```python
from build123d import *

# Parameters (mm, degrees)
SKETCH1_R           = 7.75
SKETCH1_R_2         = 1.524
BOSS_EXTRUDE1_DEPTH = 3.048
BOSS_EXTRUDE2_DEPTH = 25.4
CUT_EXTRUDE1_DEPTH  = 35.925


with BuildPart() as part:
    # Sketch1 → Boss-Extrude1 (new body)
    with BuildSketch(Plane(origin=(0, 0, 0), x_dir=(1, 0, 0), z_dir=(0, 1, 0))):
        with BuildLine():
            Line((25.4, 12.7), (25.4, -12.7))
            Line((25.4, -12.7), (22.225, -12.7))
            Line((22.225, -12.7), (3.175, -17.4625))
            Line((3.175, -17.4625), (0, -17.4625))
            ThreePointArc((0, -17.4625), (-1.398490879, -17.111633495), (-2.465718563, -16.142144397))
            Line((-2.465718563, -16.142144397), (-9.155410697, -6.097413793))
            ThreePointArc((-9.155410697, -6.097413793), (-11, 0), (-9.155410697, 6.097413793))
            Line((-9.155410697, 6.097413793), (-2.465718563, 16.142144397))
            ThreePointArc((-2.465718563, 16.142144397), (-1.398490879, 17.111633495), (0, 17.4625))
            Line((0, 17.4625), (3.175, 17.4625))
            Line((3.175, 17.4625), (22.225, 12.7))
            Line((22.225, 12.7), (25.4, 12.7))
        make_face()
        Circle(SKETCH1_R, mode=Mode.SUBTRACT)
        with Locations((0, 14.5)):
            Circle(SKETCH1_R_2, mode=Mode.SUBTRACT)
        with Locations((0, -14.5)):
            Circle(SKETCH1_R_2, mode=Mode.SUBTRACT)
    extrude(amount=BOSS_EXTRUDE1_DEPTH)

    # Sketch2 → Boss-Extrude2 (add)
    with BuildSketch(Plane(origin=(0, 3.048, 0), x_dir=(1, 0, 0), z_dir=(0, 1, 0))):
        Polygon((3.175, 17.4625), (3.175, 14.844327928), (21.912311711, 10.16), (22.86, 10.16), (22.86, -10.16), (21.912311711, -10.16), (3.175, -14.844327928), (3.175, -17.4625), (22.225, -12.7), (25.4, -12.7), (25.4, 12.7), (22.225, 12.7), align=None)
    extrude(amount=BOSS_EXTRUDE2_DEPTH)

    # Sketch3 → Cut-Extrude1 (cut, through all)
    with BuildSketch(Plane(origin=(0, 0, -17.4625), x_dir=(-1, 0, 0), z_dir=(0, 0, -1))):
        with BuildLine():
            Line((-22.225, 28.448), (-3.175, 28.448))
            Line((-3.175, 28.448), (-3.175, 3.048))
            ThreePointArc((-3.175, 3.048), (-15.471871229, 13.669096578), (-22.225, 28.448))
        make_face()
    extrude(amount=-CUT_EXTRUDE1_DEPTH, mode=Mode.SUBTRACT)


solid = part.part
```
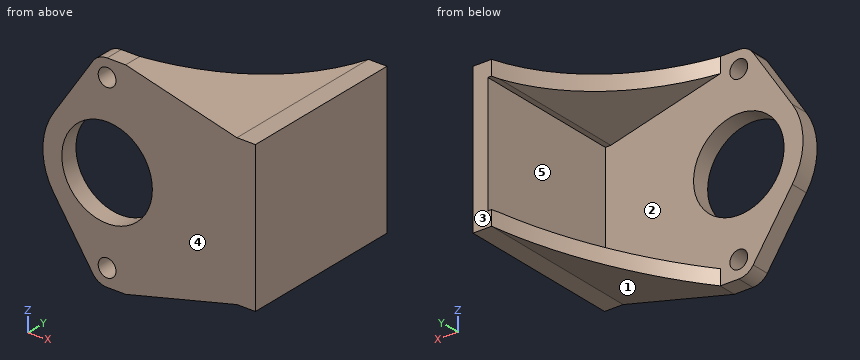
The listing builds one solid part. Answer for the finished solid, in the listing's coordinates (mm). Face numbers are marked on the shaded views. A direction names the side the tool comes from. Round coordinates to 2 decimals unless told otherwise and drop trailing zeros. Loops run counter-clockwise (first coordinate to the right, second up) from the corner with the lowest first, then second, coordinate; pieces in that order, holes last. Notation, with made-up numbers: (-38.5, -35.5) - (7.5, -35.5) arc R22 ccw to (7.5, -7.5) - close; hole circle Ø1 at (-29.75, 89). An arc over 180 degrees is marked (long way). Return JSON: item names as keys, results as strings. Group by question number.
1. Each of these flat-tipped pins is pushed along its axis until it touches: P1, Ø2, axis at x = 14.5, y = 8.5, coming from the +Z side; P2, Ø1.6, axis at x = 24, y = 15, coming from the +Z side; P3, Ø1, axis at x = -2.5, z = 9.5, coming from the +Y side. Where does it stop, or does it pass through?
2. The part is cut by section B-B on z = 0. Determine the outline of the cut face in (x, y).
3. The mould has two halves that part along Z. Classify the marked faces 1, 2 and 3: pulls with the +Z half, pulls with the -Z half, needs draft (parallel to the pull), parting line crosses it, or undercut.
4. The part is cut by section C-C on x = 7. Determine the outline of the cut face in (y, z), then the cut area to 3 significant figures.
5. Which of the six approach directions +Z, -Z, +X, -X, +Y, -Y give full straight-line access (tool end or side, diameter ignored) to the marked faces 4 and 5?
6. The part is cut by section A-A on y = 2.25. State how many separate pieces and enclosed holes the cut face has, then the cut area to 3 significant figures.
7. Consider probe 1 along Z at (x, y) = (0, 1.3); probe 2 along X at (y, z) = (1.65, 0); probe 3 along Y at (x, z) = (5, -8). Determine where each line is inside the solid, lowest interval first.
8. The part is cut by section D-D on y = 26.25. Determine the outline of the cut face in (x, z) (3 decimals).
Resolved:
{
 "1": {"P1": "stops at z = 14.88", "P2": "stops at z = 12.7", "P3": "stops at y = 3.05"},
 "2": {"outline": "(-11, 0) - (-7.75, 0) - (-7.75, 3.05) - (-11, 3.05) - close; (7.75, 0) - (25.4, 0) - (25.4, 28.45) - (22.86, 28.45) - (22.86, 3.05) - (7.75, 3.05) - close"},
 "3": {"face 1": "pulls with the -Z half", "face 2": "undercut", "face 3": "needs draft"},
 "4": {"outline": "(0, -16.51) - (5.43, -16.51) - (5.43, -13.89) - (3.05, -13.89) - (3.05, -3.33) - (0, -3.33) - close; (0, 3.33) - (3.05, 3.33) - (3.05, 13.89) - (5.43, 13.89) - (5.43, 16.51) - (0, 16.51) - close", "area": "92.8 mm²"},
 "5": {"face 4": "+Z, -Z, +X, -X, -Y", "face 5": "-X, +Y"},
 "6": {"separate pieces": "1", "enclosed holes": "3", "area": "811 mm²"},
 "7": {"probe 1": "z = -17.46 to -16.02, -12.98 to -7.75, 7.75 to 12.98, 16.02 to 17.46", "probe 2": "x = -11 to -7.75, 7.75 to 25.4", "probe 3": "y = 0 to 3.05"},
 "8": {"outline": "(21.679, -12.836) - (22.225, -12.7) - (25.4, -12.7) - (25.4, 12.7) - (22.225, 12.7) - (21.679, 12.836) - (21.679, 10.218) - (21.912, 10.16) - (22.86, 10.16) - (22.86, -10.16) - (21.912, -10.16) - (21.679, -10.218) - close"}
}
